from build123d import *

# Parameters (mm, degrees)
BOSS_EXTRUDE1_DEPTH = 57
CUT_EXTRUDE1_REACH  = 63.868


with BuildPart() as part:
    # Sketch1 → Boss-Extrude1 (new body)
    with BuildSketch(Plane(origin=(0, 0, 0), x_dir=(0, 0, -1), z_dir=(1, 0, 0))):
        Polygon((0, 0), (19.32, 0), (4.99, 14.33), (-13, 14.33), (-13, 11.33), (0, 11.33), (0, 8), (-13, 8), (-13, 5), (0, 5), align=None)
    extrude(amount=-BOSS_EXTRUDE1_DEPTH)

    # Sketch2 → Cut-Extrude1 (cut, up to next)
    with BuildSketch(Plane(origin=(0, 14.33, 0), x_dir=(1, 0, 0), z_dir=(0, 1, 0)), mode=Mode.PRIVATE) as cut_extrude1_sk1:
        Polygon((-6.5, -13), (-8.279148287, 1.49), (-48.720851713, 1.49), (-50.5, -13), align=None)
    cut_extrude1_tool1 = extrude(cut_extrude1_sk1.sketch, amount=-CUT_EXTRUDE1_REACH, mode=Mode.PRIVATE) & part.part
    add(cut_extrude1_tool1.solids().sort_by_distance((-28.5, 14.33, 5.856766))[0], mode=Mode.SUBTRACT)


solid = part.part
Could you check a few things on this model? Use its own coordinates, in mm. A direction names the side the tool comes from. Coordinates: 2 decimals unless noted, no trailing zeros. Loops run counter-clockwise (first coordinate to the right, second up) from the corner with the lowest first, then second, coordinate; pieces in that order, holes last.
1. Imagine slicing it at D-D (y = 6.5). Please give me the cut outline in (x, z).
2. I need wall thicknesses on L1, parallel to X at y = 3.75, z = -1; L2, parallel to X at y = 6.75, z = 1; L3, parallel to Z at x = -29.5, y = 11.5. Which ranges of each line are inside material? Lowest first, please.
3. We'd pull the mould along Y, two halves only. Please class faces 4 (the face through (-4, 5, 7)), 5 (the face through (0, 7, -3)), 6 (the face through (-53, 11.33, 7)), 7 (the face through (-4, 10, 0)): released by +Y, released by -Y, zero draft, split by the parting line, or undercut.
4. Imagine slicing it at B-B (z = 3). Please give me the cut outline in (x, y), and give its area (3 significant figures).
5. For P1, Ø9, axis at x = -54, z = 9, coming from the -Y side; P2, Ø7, axis at x = -31, y = 5.5, coming from the +Z side; P3, Ø1.7, axis at x = -51, y = 10, coming from the +Z side, each with a flat end and sliding along its axis, tell me the tip position at first contact or that it passes through.
6. Imagine slicing it at A-A (y = 9.5). Please give me the cut outline in (x, z), and give its area (3 significant figures).
7. For faces 1 (the face through (-53, 10, 0)), 2 (the face through (-53, 5, 7)), 3 (the face through (-49.598, 7.265, 5.654)), which set-ups out of +Z, -Z, +X, -X, +Y, -Y let a thin tool reach every point of the face, with its end or its side?
8. Imagine slicing it at C-C (z = -17). Please give me the cut outline in (x, y).
Computed values:
1. outline: (-57, -12.82) - (0, -12.82) - (0, 13) - (-6.5, 13) - (-8.28, -1.49) - (-48.72, -1.49) - (-50.5, 13) - (-57, 13) - close
2. L1: x = -57 to -48.78, -8.22 to 0
2. L2: x = -57 to -49.03, -7.97 to 0
2. L3: z = -7.82 to -1.49
3. face 4: released by -Y
3. face 5: zero draft
3. face 6: undercut
3. face 7: undercut
4. outline: (-57, 5) - (-49.27, 5) - (-49.27, 8) - (-57, 8) - close; (-57, 11.33) - (-49.27, 11.33) - (-49.27, 14.33) - (-57, 14.33) - close; (-7.73, 5) - (0, 5) - (0, 8) - (-7.73, 8) - close; (-7.73, 11.33) - (0, 11.33) - (0, 14.33) - (-7.73, 14.33) - close
4. area: 92.7 mm2
5. P1: stops at y = 5
5. P2: stops at z = -1.49
5. P3: stops at z = 0
6. outline: (-57, -9.82) - (0, -9.82) - (0, 0) - (-8.1, 0) - (-8.28, -1.49) - (-48.72, -1.49) - (-48.9, 0) - (-57, 0) - close
6. area: 499 mm2
7. face 1: +Z, +X, -X
7. face 2: +Z, +X, -X, -Y
7. face 3: +Z, +Y, -Y
8. outline: (-57, 0) - (0, 0) - (0, 2.32) - (-57, 2.32) - close
